from build123d import *

# Parameters (mm, degrees)
SKETCH1_R           = 12.7
SKETCH1_R_2         = 8.89
BOSS_EXTRUDE1_DEPTH = 266.7
SKETCH3_R           = 10.16
CUT_EXTRUDE1_DEPTH  = 12.7
CHAMFER1_SIZE       = 1.27
FILLET1_R           = 0.635


with BuildPart() as part:
    # Sketch1 → Boss-Extrude1 (new body)
    with BuildSketch(Plane.XY):
        Circle(SKETCH1_R)
        Circle(SKETCH1_R_2, mode=Mode.SUBTRACT)
    extrude(amount=BOSS_EXTRUDE1_DEPTH)

    # Sketch2 → Revolve1 (revolve)
    with BuildSketch(Plane(origin=(0, 0, 0), x_dir=(1, 0, 0), z_dir=(0, 1, 0))):
        with BuildLine():
            Line((-12.7, -266.7), (0, -266.7))
            Line((0, -266.7), (0, -279.4))
            ThreePointArc((0, -279.4), (-8.980256121, -275.680256121), (-12.7, -266.7))
        make_face()
    revolve(axis=Axis((0, 0, 279.4), (0, 0, -1)))

    # Sketch3 → Cut-Extrude1 (cut)
    with BuildSketch(Plane(origin=(0, 0, 0), x_dir=(-1, 0, 0), z_dir=(0, 0, -1))):
        Circle(SKETCH3_R)
    extrude(amount=-CUT_EXTRUDE1_DEPTH, mode=Mode.SUBTRACT)

    # Chamfer1
    chamfer1_edges = [part.edges().sort_by_distance(p)[0] for p in [
        (10.16, 0, 0),
    ]]
    chamfer(chamfer1_edges, length=CHAMFER1_SIZE)

    # Fillet1
    fillet1_edges = [part.edges().sort_by_distance(p)[0] for p in [
        (10.16, 0, 12.7),
    ]]
    fillet(fillet1_edges, radius=FILLET1_R)


solid = part.part
The listing builds one solid part. Answer for the finished solid, in the listing's coordinates (mm). Coordinates: 2 decimals unless noted, no trailing zeros. Write each loop counter-clockwise with the first axis right and the second up, starting at its lowest first coordinate (ties: lowest second). Pieces come first, ordered by that corner, then holes. Notation, with made-up numbers: M -26.5,55 L 30.5,55 A17 cw 30.5,73 Z; hole C 81.25,60.5 d9. An arc over 180 degrees is marked long. Put each result on its own line as item: value. Start each with the question number.
1. A cutting plane is placed at C-C on z = 152. Write down the section's boundary in (x, y).
2. A cutting plane is placed at A-A on y = 0. Write down the section's boundary in (x, z) (3 decimals), then the cut area to 3 significant figures.
3. Flat-ended cylindrical pins translate along their axes: P1, Ø6, axis at x = 4.5, z = 189, coming from the +Y side; P2, Ø2, axis at y = 8, z = 91, coming from the +X side; P3, Ø5.5, axis at x = 0.5, y = 1, coming from the -Z side. Find the tip coordinate at first contact, or state that the pin passes through.
4. Consider line 1 (Y direction, x = -0.25, z = 183); line 2 (Y direction, x = 0, z = 9.75). Determine where each line is inside the solid, lowest interval first. Write a range as from..to.
5. For a pull along X with two mould halves and no side action, classify faces 1 (the cylindrical face through (-2.75, -12.4, 131.48)), 2 (the cylindrical face through (-1.93, -8.68, 137.92)) as pulls with the +X half, pulls with the -X half, needs draft (parallel to the pull), parting line crosses it, or undercut.
Resolved:
1. outline: C 0,0 d25.4; hole C 0,0 d17.78
2. outline: M -12.7,0 L -11.43,0 L -10.16,1.27 L -10.16,12.065 A0.635 cw -9.525,12.7 L -8.89,12.7 L -8.89,266.7 L 8.89,266.7 L 8.89,12.7 L 9.525,12.7 A0.635 cw 10.16,12.065 L 10.16,1.27 L 11.43,0 L 12.7,0 L 12.7,266.7 A12.7 ccw -12.7,266.7 Z
2. area: 2,250 mm2
3. P1: stops at y = 12.61
3. P2: stops at x = 10.6
3. P3: stops at z = 266.7
4. line 1: y = -12.7..-8.89, 8.89..12.7
4. line 2: y = -12.7..-10.16, 10.16..12.7
5. face 1: parting line crosses it
5. face 2: undercut
